The drawing under review shows one solid part. Ordinate dimensions are in mm from its lowest x, y, z. A direction names the side the tool comes from. Give positions to 0.01 mm unless a question says otherwise; leave off trailing zeros. Loops run counter-clockwise (first coordinate to the right, second up) from the corner with the lowest first, then second, coordinate; pieces in that order, holes last. Notation, with made-up numbers: (26.5, -9) -> (41.5, -9) arc R21 ccw to (41.5, 8) -> close; hole circle Ø11 at (0.25, 67.5). An arc over 180 degrees is marked (long way). Answer in a Markdown table with one row per item. Add a question column.
(1) Consider section C-C on z = 13.5. Write out the cut boundary in (x, y), then the cut area to 3 significant figures.
(2) For line 1 (Y direction, x = 22.5, z = 26.5); line 2 (Z direction, x = 31.5, y = 10.5), list the stretches that pass through material, from the lowest coordinate up.
(3) For the marked faces 5 and 6, list the 3-axis set-ups (+Z, -Z, +X, -X, +Y, -Y) from which the entire face can be reached by the end or side of a thin tool; tool diameter is ignored.
(4) Draft analysis for pull direction Y (two halves, no side actions). For the marked faces 1, 2, 3 and 4, state which applies: +Y half, -Y half, draft (parallel to the pull), parting line (faces both ways), or undercut.
(5) Consider section D-D on y = 26. Write out the cut boundary in (x, z), then the cut area to 3 significant figures.
(6) Consider section A-A on x = 91.5. Write out the cut boundary in (y, z).
(7) Consider section B-B on y = 45. Write out the cut boundary in (x, z).
(8) For pin 1 (1.5 mm diameter, centred on x = 17.5, y = 2, fed in from +Z); pin 2 (1.5 mm diameter, centred on x = 27.5, y = 20.5, fed in from +Z); pin 3 (3 mm diameter, centred on y = 27, z = 26, fed in from +X), all flat-tipped, find the tip position at first contact; note any pin that passes through.
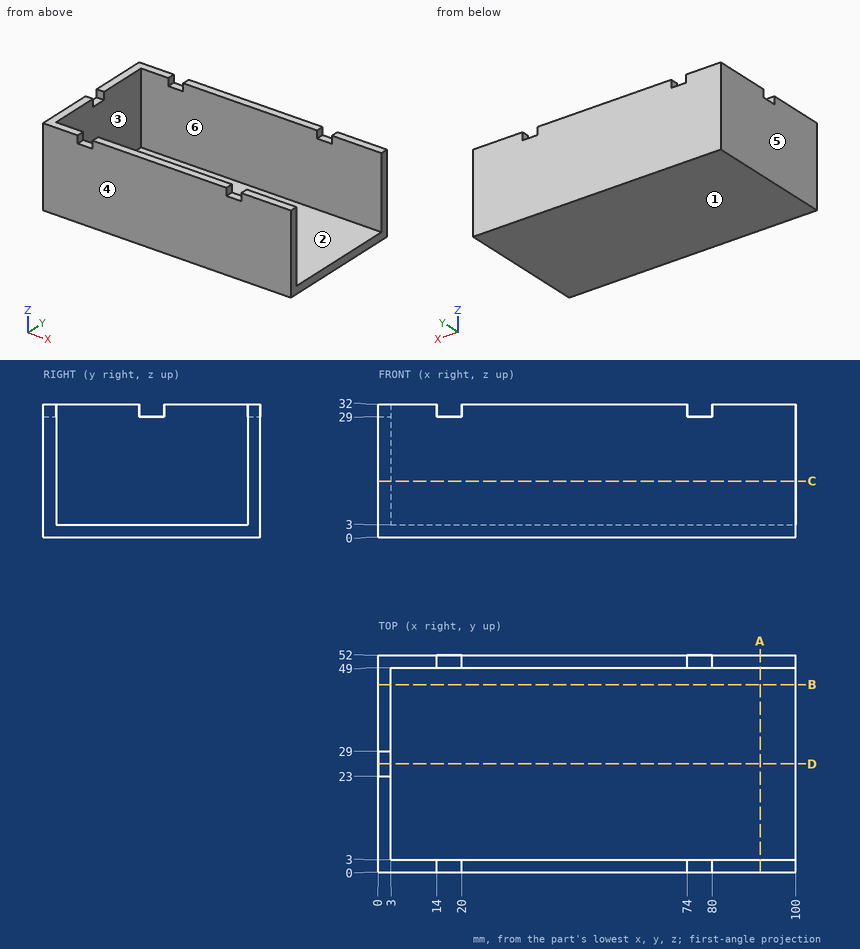
Values follow:
| question | item | result |
|---|---|---|
| 1 | outline | (0, 0) -> (100, 0) -> (100, 3) -> (3, 3) -> (3, 49) -> (100, 49) -> (100, 52) -> (0, 52) -> close |
| 1 | area | 738 mm2 |
| 2 | line 1 | 0 to 3, 49 to 52 |
| 2 | line 2 | 0 to 3 |
| 3 | face 5 | +Z, -Z, -X, +Y, -Y |
| 3 | face 6 | +Z, +X |
| 4 | face 1 | draft |
| 4 | face 2 | undercut |
| 4 | face 3 | undercut |
| 4 | face 4 | -Y half |
| 5 | outline | (0, 0) -> (100, 0) -> (100, 3) -> (3, 3) -> (3, 29) -> (0, 29) -> close |
| 5 | area | 378 mm2 |
| 6 | outline | (0, 0) -> (52, 0) -> (52, 32) -> (49, 32) -> (49, 3) -> (3, 3) -> (3, 32) -> (0, 32) -> close |
| 7 | outline | (0, 0) -> (100, 0) -> (100, 3) -> (3, 3) -> (3, 32) -> (0, 32) -> close |
| 8 | pin 1 | z = 29 |
| 8 | pin 2 | z = 3 |
| 8 | pin 3 | x = 3 |
